Autodesk Inventor part; units mm, degrees
ref_plane "YZ Plane" through (0, 0, 0) normal (1, 0, 0) x (0, 1, 0)
ref_plane "XZ Plane" through (0, 0, 0) normal (0, 1, 0) x (-1, 0, 0)
ref_plane "XY Plane" through (0, 0, 0) normal (0, 0, 1) x (1, 0, 0)
sketch "Sketch1" plane through (0, 0, 0) normal (0, 0, 1) x (1, 0, 0)
  line L0 (17.6686, 31.4113) -> (84.3436, 31.4113)
  line L1 (87.5186, 28.2363) -> (87.5186, -44.7887)
  line L2 (14.4936, -44.7887) -> (14.4936, 28.2363)
  line L3 (30.3686, 18.7113) -> (71.6436, 18.7113)
  line L4 (74.8186, 15.5363) -> (74.8186, -41.6137)
  line L5 (27.1936, 15.5363) -> (27.1936, -41.6137)
  circle A0 centre (20.8436, 25.0613) radius 2.5527
  circle A1 centre (81.1686, 25.0613) radius 2.5527
  arc A2 (17.6686, 31.4113) -> (14.4936, 28.2363) centre (17.6686, 28.2363) ccw
  arc A3 (87.5186, 28.2363) -> (84.3436, 31.4113) centre (84.3436, 28.2363) ccw
  circle A4 centre (20.8436, -38.4387) radius 2.5527
  circle A5 centre (81.1686, -38.4387) radius 2.5527
  line L6 (30.3686, -44.7887) -> (71.6436, -44.7887)
  line L7 (87.5186, -44.7887) -> (87.5186, -79.7137)
  line L8 (84.3436, -82.8887) -> (17.6686, -82.8887)
  line L9 (14.4936, -79.7137) -> (14.4936, -44.7887)
  circle A6 centre (51.0061, -63.8387) radius 6.35
  arc A7 (14.4936, -79.7137) -> (17.6686, -82.8887) centre (17.6686, -79.7137) ccw
  arc A8 (84.3436, -82.8887) -> (87.5186, -79.7137) centre (84.3436, -79.7137) ccw
  arc A9 (71.6436, -44.7887) -> (74.8186, -41.6137) centre (71.6436, -41.6137) ccw
  arc A10 (27.1936, -41.6137) -> (30.3686, -44.7887) centre (30.3686, -41.6137) ccw
  arc A11 (30.3686, 18.7113) -> (27.1936, 15.5363) centre (30.3686, 15.5363) ccw
  arc A12 (74.8186, 15.5363) -> (71.6436, 18.7113) centre (71.6436, 15.5363) ccw
  point P0 (0, 0)
  point P1 (87.5186, 31.4113)
  dimension "d1" = 76.2
  dimension "d2" = 73.025
  dimension "d3" = 12.7
  dimension "d4" = 12.7
  dimension "d5" = 12.7
  dimension "d6" = 5.1054
  dimension "d7" = 6.35
  dimension "d9" = 5.1054
  dimension "d10" = 6.35
  dimension "d11" = 6.35
  dimension "d12" = 3.175
  dimension "d13" = 5.1054
  dimension "d14" = 5.1054
  dimension "d15" = 63.5
  dimension "d16" = 63.5
  dimension "d17" = 76.2
  dimension "d18" = 12.7
  dimension "d19" = 36.5125
  dimension "d20" = 38.1
  dimension "d21" = 19.05
  dimension "d22" = 3.175
  dimension "d23" = 3.175
  dimension "d26" = 60.325
  dimension "d27" = 0
extrude "Extrusion1" add sketch "Sketch1" along normal blind 6.35
properties part number "2 Stage Climber in a box bracket"
Here's how the part is built. I have some questions about the finished solid (model axes, mm). A direction names the side the tool comes from. Coordinates: 2 decimals unless noted, no trailing zeros. Order: outer loops, then holes, each group sorted by start corner. A loop starts at its lowest first (then second) coordinate and runs counter-clockwise, first axis right, second up.
1) Imagine slicing it at A-A on y = -25. List the corners of the cut face in (x, z) for me, and give its area (3 significant figures).
2) Which directions (+Z, -Z, +X, -X, +Y, -Y) give clear straight access to the entire face, cutting with the end or side of a thin tool? Please do faces 4 (the face through (51, -44.789, 3)), 5 (the face through (51, -82.889, 3)).
3) We'd pull the mould along X, two halves only. Please class faces 1 (the face through (28.1, 17.76, 3.13)), 2 (the face through (15.4, 30.46, 3.13)), 3 (the face through (86.56, 30.51, 3.13)): +X half, -X half, draft (parallel to the pull), parting line (faces both ways), or undercut.
4) Imagine slicing it at B-B on x = 68.5. List the corners of the cut face in (y, z) for me.
5) Imagine slicing it at C-C on x = 56. List the corners of the cut face in (y, z) for me.
6) Imagine slicing it at D-D on z = 5. List the corners of the cut face in (x, y) for me (3 decimals).
7) I need wall thicknesses on line 1 (X direction, y = 25, z = 4.5); line 2 (Y direction, x = 64.5, z = 2.75); line 3 (Y direction, x = 23, z = 3). Which ranges of each line are inside material? Lowest first, please.
Response values:
1. outline: (14.49, 0) - (27.19, 0) - (27.19, 6.35) - (14.49, 6.35) - close; (74.82, 0) - (87.52, 0) - (87.52, 6.35) - (74.82, 6.35) - close
1. area: 161 mm2
2. face 4: +Z, -Z
2. face 5: +Z, -Z, +X, -X, -Y
3. face 1: undercut
3. face 2: -X half
3. face 3: +X half
4. outline: (-82.89, 0) - (-44.79, 0) - (-44.79, 6.35) - (-82.89, 6.35) - close; (18.71, 0) - (31.41, 0) - (31.41, 6.35) - (18.71, 6.35) - close
5. outline: (-82.89, 0) - (-67.76, 0) - (-67.76, 6.35) - (-82.89, 6.35) - close; (-59.92, 0) - (-44.79, 0) - (-44.79, 6.35) - (-59.92, 6.35) - close; (18.71, 0) - (31.41, 0) - (31.41, 6.35) - (18.71, 6.35) - close
6. outline: (14.494, -79.714) arc R3.175 ccw to (17.669, -82.889) - (84.344, -82.889) arc R3.175 ccw to (87.519, -79.714) - (87.519, 28.236) arc R3.175 ccw to (84.344, 31.411) - (17.669, 31.411) arc R3.175 ccw to (14.494, 28.236) - close; hole circle Ø5.105 at (20.844, -38.439); hole circle Ø5.105 at (20.844, 25.061); hole (27.194, -41.614) arc R3.175 ccw to (30.369, -44.789) - (71.644, -44.789) arc R3.175 ccw to (74.819, -41.614) - (74.819, 15.536) arc R3.175 ccw to (71.644, 18.711) - (30.369, 18.711) arc R3.175 ccw to (27.194, 15.536) - close; hole circle Ø12.7 at (51.006, -63.839); hole circle Ø5.105 at (81.169, -38.439); hole circle Ø5.105 at (81.169, 25.061)
7. line 1: x = 14.49 to 18.29, 23.4 to 78.62, 83.72 to 87.52
7. line 2: y = -82.89 to -44.79, 18.71 to 31.41
7. line 3: y = -82.89 to -39.8, -37.07 to 23.7, 26.43 to 31.41
